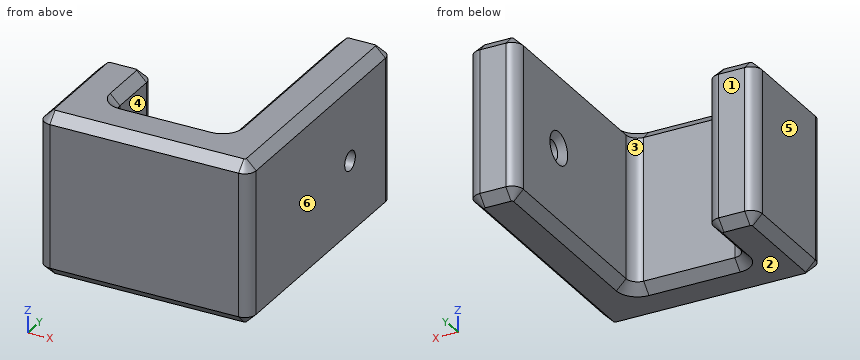
```python
from build123d import *

# Parameters (mm, degrees)
PAD_DEPTH       = 50
CHAMFER_SIZE    = 3
CHAMFER001_SIZE = 3
SKETCH001_R     = 3
POCKET_DEPTH    = 15.11578
CHAMFER002_SIZE = 2


with BuildPart() as part:
    # Sketch → Pad (new body)
    with BuildSketch(Plane.XY):
        with BuildLine():
            Line((-35.88522, 9.618171), (-35.88522, -20.381829))
            ThreePointArc((-35.88522, -20.381829), (-34.860094, -22.856703), (-32.38522, -23.881829))
            Line((-32.38522, -23.881829), (25.61478, -23.881829))
            ThreePointArc((25.61478, -23.881829), (28.089653, -22.856703), (29.11478, -20.381829))
            Line((29.11478, -20.381829), (29.11478, 52.618171))
            ThreePointArc((29.11478, 52.618171), (28.089653, 55.093044), (25.61478, 56.118171))
            Line((25.61478, 56.118171), (17.61478, 56.118171))
            ThreePointArc((17.61478, 56.118171), (15.139906, 55.093044), (14.11478, 52.618171))
            Line((14.11478, 52.618171), (14.11478, -5.381829))
            ThreePointArc((10.61478, -8.881829), (13.089653, -7.856703), (14.11478, -5.381829))
            Line((10.61478, -8.881829), (-17.38522, -8.881829))
            ThreePointArc((-20.88522, -5.381829), (-19.860094, -7.856703), (-17.38522, -8.881829))
            Line((-20.88522, -5.381829), (-20.88522, 9.618171))
            ThreePointArc((-20.88522, 9.618171), (-21.910347, 12.093044), (-24.38522, 13.118171))
            Line((-24.38522, 13.118171), (-32.38522, 13.118171))
            ThreePointArc((-32.38522, 13.118171), (-34.860094, 12.093044), (-35.88522, 9.618171))
        make_face()
    extrude(amount=PAD_DEPTH)

    # Chamfer
    chamfer_edges = [part.edges().sort_by_distance(p)[0] for p in [
        (29.11478, 16.118171, 0),
    ]]
    chamfer(chamfer_edges, length=CHAMFER_SIZE)

    # Chamfer001
    chamfer001_edges = [part.edges().sort_by_distance(p)[0] for p in [
        (29.11478, 16.118171, 50),
    ]]
    chamfer(chamfer001_edges, length=CHAMFER001_SIZE)

    # Sketch001 (on DatumPlane) → Pocket (cut, through all)
    with BuildSketch(Plane(origin=(14, 0, 0), x_dir=(0, 0, -1), z_dir=(1, 0, 0))):
        with Locations((-25, 32.618171)):
            Circle(SKETCH001_R)
    extrude(amount=POCKET_DEPTH, mode=Mode.SUBTRACT)

    # Chamfer002
    chamfer002_edges = [part.edges().sort_by_distance(p)[0] for p in [
        (14.11478, 32.618171, 28),
    ]]
    chamfer(chamfer002_edges, length=CHAMFER002_SIZE)


solid = part.part
```
For this review, take the finished solid that the model builds, in its own axes (mm). Face numbers are marked on the shaded views. A direction names the side the tool comes from. Round coordinates to 2 decimals unless told otherwise and drop trailing zeros. Write each loop counter-clockwise with the first axis right and the second up, starting at its lowest first coordinate (ties: lowest second). Pieces come first, ordered by that corner, then holes. Notation, with made-up numbers: (14.25, 5.5) - (21.25, 5.5) arc R17 ccw to (21.25, 28.5) - close; hole circle Ø6 at (9, 39). An arc over 180 degrees is marked (long way). Write each question's results on one line, items separated by ' | '.
Item 1: Draft analysis for pull direction X (two halves, no side actions). For the marked faces 4, 5 and 6, state which applies: pulls with the +X half, pulls with the -X half, needs draft (parallel to the pull), parting line crosses it, or undercut.
Calculated:
face 4: undercut | face 5: pulls with the -X half | face 6: pulls with the +X half
Item 2: To check wall thickness, follow line 1 along X through (y, z) = (-5, 22.5); line 2 along Y through (x, z) = (25, 25); line 3 along X through (y, z) = (44.5, 42). State the ranges of each line that lie inside material, in increasing order. Write a range as from..to.
Calculated:
line 1: x = -35.89..-20.89, 14.11..29.11 | line 2: y = -23.88..29.62, 35.62..56.12 | line 3: x = 14.11..29.11
Item 3: For the marked faces 1, 2 and 3, list the 3-axis set-ups (+Z, -Z, +X, -X, +Y, -Y) from which the entire face can be reached by the end or side of a thin tool; tool diameter is ignored.
Calculated:
face 1: +Z, -Z, -X, +Y | face 2: -Z, +X, -X, +Y, -Y | face 3: +Z, -Z, +Y
Item 4: Take a section at A-A on z = 25. State the section outline as (x, y) points, then the cut area to 3 significant figures.
Calculated:
outline: (-35.89, -20.38) arc R3.5 ccw to (-32.39, -23.88) - (25.61, -23.88) arc R3.5 ccw to (29.11, -20.38) - (29.11, 29.62) - (16.11, 29.62) - (14.11, 27.62) - (14.11, -5.38) arc R3.5 cw to (10.61, -8.88) - (-17.39, -8.88) arc R3.5 cw to (-20.89, -5.38) - (-20.89, 9.62) arc R3.5 ccw to (-24.39, 13.12) - (-32.39, 13.12) arc R3.5 ccw to (-35.89, 9.62) - close; (14.11, 37.62) - (16.11, 35.62) - (29.11, 35.62) - (29.11, 52.62) arc R3.5 ccw to (25.61, 56.12) - (17.61, 56.12) arc R3.5 ccw to (14.11, 52.62) - close | area: 2,180 mm^2
Item 5: Take a section at B-B on x = -0.5. State the section outline as (y, z) points.
Calculated:
outline: (-23.88, 3) - (-20.88, 0) - (-11.88, 0) - (-8.88, 3) - (-8.88, 47) - (-11.88, 50) - (-20.88, 50) - (-23.88, 47) - close
Item 6: For pin 1 (22.5 mm diameter, centred on x = 1, z = 23, fed in from +Y); pin 2 (9.5 mm diameter, centred on y = 32.62, z = 25, fed in from -X); pin 3 (6.5 mm diameter, centred on x = -29.5, z = 33.5, fed in from +Y), all flat-tipped, find the tip position at first contact; note any pin that passes through.
Calculated:
pin 1: stops at y = -8.48 | pin 2: stops at x = 14.36 | pin 3: stops at y = 13.12
Item 7: Take a section at C-C on y = 20.5. State the section outline as (x, z) points, then the cut area to 3 significant figures.
Calculated:
outline: (14.11, 3) - (17.11, 0) - (26.11, 0) - (29.11, 3) - (29.11, 47) - (26.11, 50) - (17.11, 50) - (14.11, 47) - close | area: 732 mm^2
Item 8: Take a section at D-D on z = 41.5. State the section outline as (x, y) points.
Calculated:
outline: (-35.89, -20.38) arc R3.5 ccw to (-32.39, -23.88) - (25.61, -23.88) arc R3.5 ccw to (29.11, -20.38) - (29.11, 52.62) arc R3.5 ccw to (25.61, 56.12) - (17.61, 56.12) arc R3.5 ccw to (14.11, 52.62) - (14.11, -5.38) arc R3.5 cw to (10.61, -8.88) - (-17.39, -8.88) arc R3.5 cw to (-20.89, -5.38) - (-20.89, 9.62) arc R3.5 ccw to (-24.39, 13.12) - (-32.39, 13.12) arc R3.5 ccw to (-35.89, 9.62) - close
